from build123d import *

# Parameters (mm, degrees)
BOSS_EXTRUDE1_DEPTH         = 15.875
TAP_DRILL_FOR_1_4_20_TAP1_D = 5.1054
CHAMFER1_SIZE               = 0.254


with BuildPart() as part:
    # Model → Boss-Extrude1 (new body)
    with BuildSketch(Plane.XY):
        with BuildLine():
            Line((15.773627649, 23.305847831), (25.584064841, 23.305847831))
            ThreePointArc((25.584064841, 23.305847831), (25.812010792, 23.16410193), (25.785700673, 22.896970812))
            Line((25.785700673, 22.896970812), (23.09847623, 19.394911734))
            ThreePointArc((23.09847623, 19.394911734), (20.678846245, 18.201682274), (18.25921626, 19.394911734))
            Line((18.25921626, 19.394911734), (15.571991817, 22.896970812))
            ThreePointArc((15.571991817, 22.896970812), (15.545681698, 23.16410193), (15.773627649, 23.305847831))
        make_face()
    extrude(amount=BOSS_EXTRUDE1_DEPTH)

    # Tap Drill for 1/4-20 Tap1 (through all)
    with Locations(Plane(origin=(0, 23.305847831, 0), x_dir=(1, 0, 0), z_dir=(0, 1, 0))):
        with Locations((20.678846245, -10.795)):
            Hole(TAP_DRILL_FOR_1_4_20_TAP1_D / 2)

    # Chamfer1
    chamfer1_edges = [part.edges().sort_by_distance(p)[0] for p in [
        (23.231546245, 23.305847831, 10.795),
    ]]
    chamfer(chamfer1_edges, length=CHAMFER1_SIZE)


solid = part.part
Work out the finished part from the listing and answer in its coordinate system (mm). Round coordinates to 2 decimals unless told otherwise and drop trailing zeros. Write each loop counter-clockwise with the first axis right and the second up, starting at its lowest first coordinate (ties: lowest second). Pieces come first, ordered by that corner, then holes.
1) A cutting plane is placed at C-C (z = 4.5). Give the vertices of the cut face in (x, y), plus the area to 3 significant figures.
2) Straight lines are drawn through the part: line 1 (X direction, y = 22.3, z = 10); line 2 (Z direction, x = 19.5, y = 20.75) (3 decimals); line 3 (Z direction, x = 21.25, y = 20.3) (3 decimals). For each, find the intervals that lie inside material, in ascending order.
3) Given pin 1 Ø3 at (y, z) = (21, 7.5) entering from -X, flat-ended and moving along its own axis, determine where the tip first touches the part or whether it passes through.
4) The mould has two halves that part along X. Classify faces 1 (the flat face through (16.934, 21.121, 7.826)), 2 (the cylindrical face through (20.7, 18.2, 4.9)), 3 (the cylindrical face through (23.23, 21.13, 10.68)): pulls with the +X half, pulls with the -X half, needs draft (parallel to the pull), parting line crosses it, or undercut.
5) A cutting plane is placed at D-D (x = 16). Give the vertices of the cut face in (y, z) (3 decimals).
6) A cutting plane is placed at B-B (y = 20.5). Give the vertices of the cut face in (x, z) (3 decimals).
7) A cutting plane is placed at A-A (y = 18.95). Give the vertices of the cut face in (x, z) (3 decimals), plus the area to 3 significant figures.
Completed:
1. outline: (15.57, 22.9) - (18.26, 19.39) arc R3.05 ccw to (23.1, 19.39) - (25.79, 22.9) arc R0.25 ccw to (25.58, 23.31) - (15.77, 23.31) arc R0.25 ccw to start
1. area: 34.6 mm2
2. line 1: x = 16.03 to 18.25, 23.1 to 25.33
2. line 2: z = 0 to 8.531, 13.059 to 15.875
2. line 3: z = 0 to 8.307, 13.283 to 15.875
3. pin 1: stops at x = 15.88
4. face 1: pulls with the -X half
4. face 2: parting line crosses it
4. face 3: undercut
5. outline: (22.339, 0) - (23.306, 0) - (23.306, 15.875) - (22.339, 15.875) - close
6. outline: (17.411, 0) - (23.946, 0) - (23.946, 15.875) - (17.411, 15.875) - close; hole circle Ø5.105 at (20.679, 10.795)
7. outline: (18.678, 0) - (22.68, 0) - (22.68, 9.21) arc R2.553 cw to (18.678, 9.21) - close; (18.678, 12.38) arc R2.553 cw to (22.68, 12.38) - (22.68, 15.875) - (18.678, 15.875) - close
7. area: 45.5 mm2
